Geometry check sheet. Reference: the model listing, model coordinates, mm. Face numbers are marked on the shaded views. A direction names the side the tool comes from. Give positions to 0.01 mm unless a question says otherwise; leave off trailing zeros. Order: outer loops, then holes, each group sorted by start corner. A loop starts at its lowest first (then second) coordinate and runs counter-clockwise, first axis right, second up. Notation, with made-up numbers: M 53,83.5 L 107,83.5 A22 ccw 107,108.5 Z; hole C 73,71 d3. An arc over 180 degrees is marked long. Answer as CSV lines item,"result". Start each with the question number.
Q1. Section check A-A, the plane y = 11. Record the boundary of the cut face in (x, z), then the cut area to 3 significant figures.
Q2. Section check D-D, the plane z = 11.75. Record the boundary of the cut face in (x, y).
Q3. Thickness scan on line 1 (Z direction, x = 2.05, y = 5.75); line 2 (X direction, y = 14, z = 10); line 3 (Y direction, x = 1.4, z = 2.75). Record the ranges inside material, lowest first.
Q4. Section check B-B, the plane z = 6.25. Record the boundary of the cut face in (x, y), then the cut area to 3 significant figures.
Q5. Set-up check for the marked faces 1, 2, 3, 4 and 5: record each of +Z, -Z, +X, -X, +Y, -Y from which the full face is reachable in a straight line by a thin tool's end or side.
Q6. Section check C-C, the plane x = 5.2. Record the boundary of the cut face in (y, z).
Q7. Go/stop test with a flat-tipped pin: pin 1 (1.7 mm diameter, centred on x = 5, y = 9.5, fed in from +Z). Record where the tip stops, or that it passes through.
```python
from build123d import *

# Parameters (mm, degrees)
EXTRUSION1_DEPTH = 12
EXTRUSION2_DEPTH = 1
CONG_3_R         = 1
CONG_4_R         = 1
CONG_5_R         = 1


with BuildPart() as part:
    # Esquisse1 → Extrusion1 (new body)
    with BuildSketch(Plane.XY):
        Polygon((0, 0), (0, 13), (3, 15.939387691), (6, 13), (6, 0), align=None)
    extrude(amount=EXTRUSION1_DEPTH)

    # Esquisse3 → Extrusion2 (add)
    with BuildSketch(Plane.XY.offset(12)):
        Polygon((2.160028245, 15.116386813), (2.160028245, 0), (3.839971755, 0), (3.839971755, 15.116386813), (3, 15.939387691), align=None)
    extrude(amount=EXTRUSION2_DEPTH)

    # Congé3
    cong_3_edges = [part.edges().sort_by_distance(p)[0] for p in [
        (1.080014123, 0, 12),
    ]]
    fillet(cong_3_edges, radius=CONG_3_R)

    # Congé4
    cong_4_edges = [part.edges().sort_by_distance(p)[0] for p in [
        (4.919985877, 0, 12),
    ]]
    fillet(cong_4_edges, radius=CONG_4_R)

    # Congé5
    cong_5_edges = [part.edges().sort_by_distance(p)[0] for p in [
        (3, 0, 13),
    ]]
    fillet(cong_5_edges, radius=CONG_5_R)


solid = part.part
```
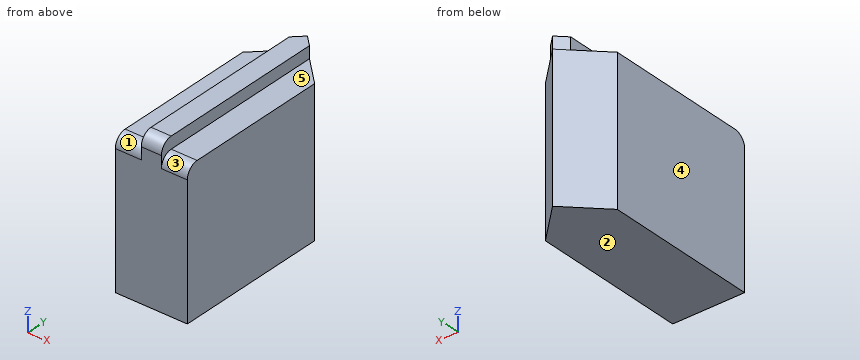
Answer block:
1,outline,"M 0,0 L 6,0 L 6,12 L 3.84,12 L 3.84,13 L 2.16,13 L 2.16,12 L 0,12 Z"
1,area,"73.7 mm2"
2,outline,"M 0,0.34 L 2.16,0.34 L 2.16,0 L 3.84,0 L 3.84,0.34 L 6,0.34 L 6,13 L 3,15.94 L 0,13 Z"
3,line 1,"z = 0 to 12"
3,line 2,"x = 1.02 to 4.98"
3,line 3,"y = 0 to 14.37"
4,outline,"M 0,0 L 6,0 L 6,13 L 3,15.94 L 0,13 Z"
4,area,"86.8 mm2"
5,face 1,"+Z, -X, -Y"
5,face 2,"-Z, +X, -X, +Y, -Y"
5,face 3,"+Z, +X, -Y"
5,face 4,"+Z, -Z, -X, +Y, -Y"
5,face 5,"+Z, +X, +Y, -Y"
6,outline,"M 0,0 L 13.78,0 L 13.78,12 L 1,12 A1 ccw 0,11 Z"
7,pin 1,"stops at z = 12"
